Geometry check sheet. Reference: the model listing, model coordinates, mm. Round coordinates to 2 decimals unless told otherwise and drop trailing zeros. Write each loop counter-clockwise with the first axis right and the second up, starting at its lowest first coordinate (ties: lowest second). Pieces come first, ordered by that corner, then holes. Notation, with made-up numbers: (-27.75, -39) -> (-0.75, -39) arc R28 cw to (-0.75, -15) -> close; hole circle Ø4 at (67, -18). An arc over 180 degrees is marked (long way). Use a Markdown table: item, result.
```python
from build123d import *

# Parameters (mm, degrees)
FASE1_SIZE = 0.5


with BuildPart() as part:
    # Skizze1 → Rotation1 (revolve)
    with BuildSketch(Plane(origin=(0, 0, 0), x_dir=(0, 0, -1), z_dir=(1, 0, 0))):
        Polygon((0, 0), (-2, 0), (-2, -30), (-2.1, -30), (-2.1, -54), (-1.5, -54), (-1.5, -184), (-2.1, -184), (-2.1, -208), (-2, -208), (-2, -238), (0, -238), align=None)
    revolve(axis=Axis((0, 0, 0), (0, 1, 0)))

    # Fase1
    fase1_edges = [part.edges().sort_by_distance(p)[0] for p in [
        (0, 0, -2),
        (0, -238, -2),
    ]]
    chamfer(fase1_edges, length=FASE1_SIZE)


solid = part.part
```
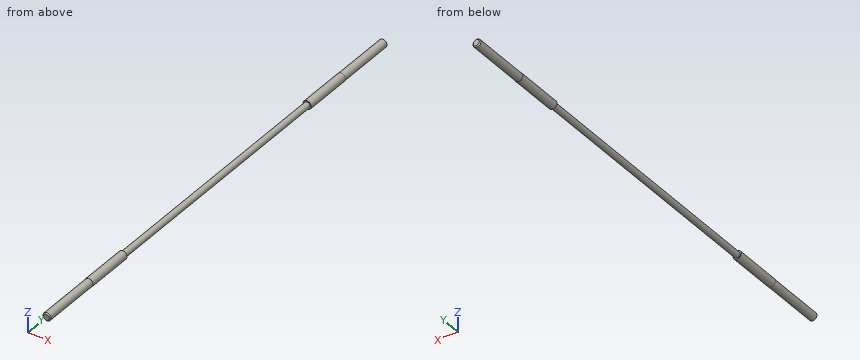
(1) Gauge pin test, flat ends, axial feed: pin 1 Ø2 at (x, y) = (0, -84.5) entering from -Z; pin 2 Ø1 at (x, y) = (1, -73) entering from -Z; pin 3 Ø2 at (y, z) = (-118, -1.5) entering from +X. Record the tip position at first contact, or that the pin passes through.
A:
| item | result |
|---|---|
| pin 1 | stops at z = -1.5 |
| pin 2 | stops at z = -1.41 |
| pin 3 | stops at x = 1.41 |
(2) Thickness scan on line 1 (Y direction, x = 1.7, z = -0.2); line 2 (Y direction, x = 0.25, z = -1.8); line 3 (Z direction, x = -0.2, y = -189). Record the ranges inside material, lowest first.
A:
| item | result |
|---|---|
| line 1 | y = -237.79 to -184, -54 to -0.21 |
| line 2 | y = -237.68 to -184, -54 to -0.32 |
| line 3 | z = -2.09 to 2.09 |
(3) Section check C-C on y = -156.5. Record the cut outline in (x, z).
A:
| item | result |
|---|---|
| outline | circle Ø3 at (0, 0) |
(4) Section check B-B on z = 0. Record the cut outline in (x, y), plus the area to 3 significant figures.
A:
| item | result |
|---|---|
| outline | (-2.1, -208) -> (-2, -208) -> (-2, -237.5) -> (-1.5, -238) -> (1.5, -238) -> (2, -237.5) -> (2, -208) -> (2.1, -208) -> (2.1, -184) -> (1.5, -184) -> (1.5, -54) -> (2.1, -54) -> (2.1, -30) -> (2, -30) -> (2, -0.5) -> (1.5, 0) -> (-1.5, 0) -> (-2, -0.5) -> (-2, -30) -> (-2.1, -30) -> (-2.1, -54) -> (-1.5, -54) -> (-1.5, -184) -> (-2.1, -184) -> close |
| area | 831 mm2 |
(5) Section check A-A on x = 0. Record the cut outline in (y, z), plus the area to 3 significant figures.
A:
| item | result |
|---|---|
| outline | (-238, -1.5) -> (-237.5, -2) -> (-208, -2) -> (-208, -2.1) -> (-184, -2.1) -> (-184, -1.5) -> (-54, -1.5) -> (-54, -2.1) -> (-30, -2.1) -> (-30, -2) -> (-0.5, -2) -> (0, -1.5) -> (0, 1.5) -> (-0.5, 2) -> (-30, 2) -> (-30, 2.1) -> (-54, 2.1) -> (-54, 1.5) -> (-184, 1.5) -> (-184, 2.1) -> (-208, 2.1) -> (-208, 2) -> (-237.5, 2) -> (-238, 1.5) -> close |
| area | 831 mm2 |
